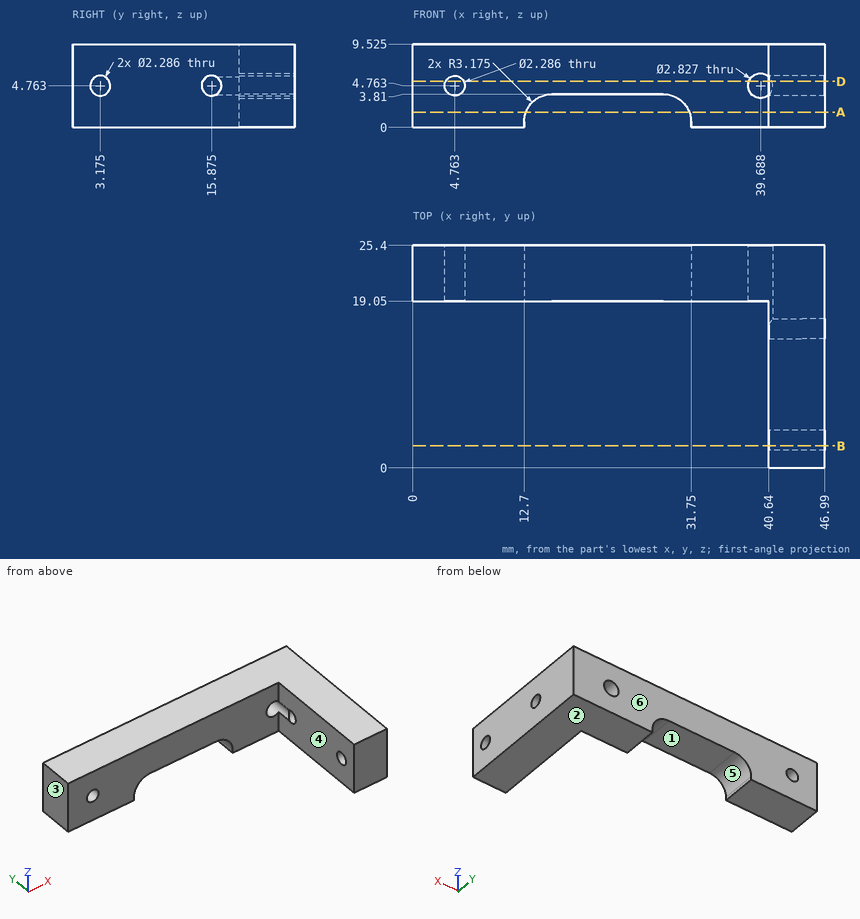
Answer from the drawing. Dimensions are ordinates in mm from the lowest x, y and z of the part. A direction names the side the tool comes from. Give positions to 0.01 mm unless a question says otherwise; leave off trailing zeros. Write each loop counter-clockwise with the first axis right and the second up, starting at its lowest first coordinate (ties: lowest second). Pieces come first, ordered by that corner, then holes. Notation, with made-up numbers: (27.25, 55.5) -> (52.25, 55.5) arc R25 ccw to (52.25, 87.5) -> close; hole circle Ø10 at (89, 81). An arc over 180 degrees is marked (long way). Use a Markdown table: item, result.
(1) Flat-ended cylindrical pins translate along their axes: P1, Ø3.5, axis at x = 4.76, z = 4.76, coming from the +Y side; P2, Ø4, axis at x = 16.5, y = 22, coming from the -Z side; P3, Ø3.5, axis at y = 3.18, z = 4.76, coming from the -X side; P4, Ø5, axis at x = 25.5, z = 4, coming from the -Y side. Find the tip coordinate at first contact, or state that the pin passes through.
Return value:
| item | result |
|---|---|
| P1 | y = 25.4 |
| P2 | z = 3.5 |
| P3 | x = 40.64 |
| P4 | y = 19.05 |
(2) Find the intervals of material crossed by probe 1 along Y at (x, z) = (45.5, 4.75); probe 2 along Z at (x, y) = (19.5, 20) (1 decimal); probe 3 along X at (y, z) = (2.5, 3), in increasing order. Write a range as from..to.
Return value:
| item | result |
|---|---|
| probe 1 | 0..2.03, 4.32..14.73, 17.02..25.4 |
| probe 2 | 3.8..9.5 |
| probe 3 | 40.64..46.99 |
(3) Section D-D, the plane z = 5.25 is taken. Give the number of separate pieces and of enclosed holes in the cut face, then the cut area to 3 significant figures.
Return value:
| item | result |
|---|---|
| separate pieces | 5 |
| enclosed holes | 0 |
| area | 362 mm2 |
(4) For the marked faces 4, 5 and 6, determine the directions among +Z, -Z, +X, -X, +Y, -Y from which every point of the face is accessible in a straight line to the end or side of a thin tool.
Return value:
| item | result |
|---|---|
| face 4 | +Z, -Z, -X, -Y |
| face 5 | -Z, +Y, -Y |
| face 6 | +Z, -Z, +X, -X, +Y |
(5) Section B-B, the plane y = 2.5 is taken. Determine the outline of the cut face in (x, z) (1 decimal).
Return value:
| item | result |
|---|---|
| outline | (40.6, 0) -> (47, 0) -> (47, 3.8) -> (40.6, 3.8) -> close; (40.6, 5.7) -> (47, 5.7) -> (47, 9.5) -> (40.6, 9.5) -> close |
(6) Determine the mould class of the marked faces 1, 2 and 3 for opening direction X: released by +X, released by -X, zero draft, split by the parting line, or undercut.
Return value:
| item | result |
|---|---|
| face 1 | undercut |
| face 2 | zero draft |
| face 3 | released by -X |
(7) Section A-A, the plane z = 1.75 is taken. Determine the outline of the cut face in (x, y), then the cut area to 3 significant figures.
Return value:
| item | result |
|---|---|
| outline | (0, 19.05) -> (12.9, 19.05) -> (12.9, 25.4) -> (0, 25.4) -> close; (31.55, 19.05) -> (40.64, 19.05) -> (40.64, 0) -> (46.99, 0) -> (46.99, 25.4) -> (31.55, 25.4) -> close |
| area | 301 mm2 |
